Print and shaded views of the part. All mm, measured from the part's lowest x, y and z. Coordinates: 2 decimals unless noted, no trailing zeros. Order: outer loops, then holes, each group sorted by start corner. A loop starts at its lowest first (then second) coordinate and runs counter-clockwise, first axis right, second up.
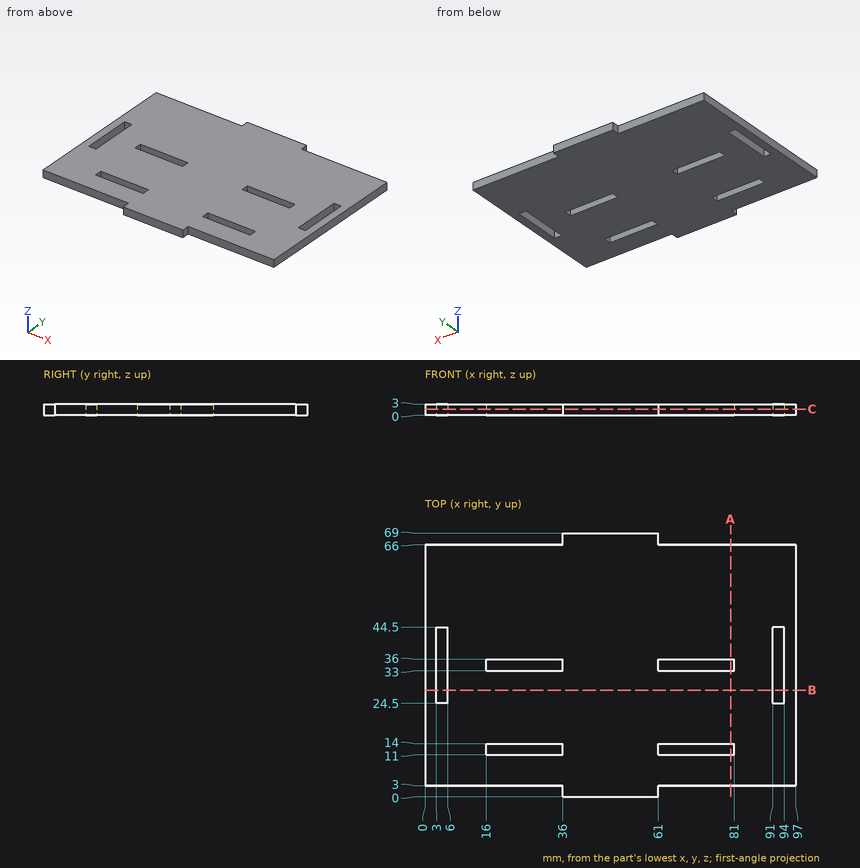
Q1. Cut at A-A, the plane x = 80. List the corners of the cut face in (y, z), plus the area to 3 significant figures.
Established:
outline: (3, 0) - (11, 0) - (11, 3) - (3, 3) - close; (14, 0) - (33, 0) - (33, 3) - (14, 3) - close; (36, 0) - (66, 0) - (66, 3) - (36, 3) - close
area: 171 mm2
Q2. Drop flat-ended pins along their axis: P1, Ø1.5, axis at x = 70.5, z = 2, coming from the +Y side; P2, Ø6, axis at x = 52.5, y = 46.5, coming from the -Z side; P3, Ø1.5, axis at y = 68, z = 1.5, coming from the +X side; P4, Ø1.5, axis at x = 85, z = 1.5, coming from the -Y side. Give the stop position or say it passes through.
Established:
P1: stops at y = 66
P2: stops at z = 0
P3: stops at x = 61
P4: stops at y = 3
Q3. Probe line 1 (Y direction, x = 23, z = 2.7); line 2 (X direction, y = 32.5, z = 1.1). List the from-to ranges inside material, lowest first.
Established:
line 1: y = 3 to 11, 14 to 33, 36 to 66
line 2: x = 0 to 3, 6 to 91, 94 to 97
Q4. Cut at B-B, the plane y = 28. List the corners of the cut face in (x, z), plus the area to 3 significant figures.
Established:
outline: (0, 0) - (3, 0) - (3, 3) - (0, 3) - close; (6, 0) - (91, 0) - (91, 3) - (6, 3) - close; (94, 0) - (97, 0) - (97, 3) - (94, 3) - close
area: 273 mm2
Q5. Cut at C-C, the plane z = 1.65. Count the separate pieces of the cut face and the enclosed holes in it, plus the area to 3 significant figures.
Established:
separate pieces: 1
enclosed holes: 6
area: 5,900 mm2
